The listing builds one solid part. Answer for the finished solid, in the listing's coordinates (mm). A direction names the side the tool comes from. Round coordinates to 2 decimals unless told otherwise and drop trailing zeros. Write each loop counter-clockwise with the first axis right and the second up, starting at its lowest first coordinate (ties: lowest second). Pieces come first, ordered by that corner, then holes. Notation, with made-up numbers: (86, 66) - (131, 66) arc R20 ccw to (131, 100) - close; hole circle Ø11 at (16, 6.5). An arc over 180 degrees is marked (long way). Answer in a Markdown table with one row per item.
from build123d import *

# Parameters (mm, degrees)
BOSS_EXTRUDE3_DEPTH   = 8
BOSS_EXTRUDE3_2_DEPTH = 8
SKETCH4_W             = 11
SKETCH4_H             = 10.5
BOSS_EXTRUDE4_DEPTH   = 2
FILLET3_R             = 3
MIRROR2_START         = -2
MIRROR2_DEPTH         = 10
MIRROR2_2_DEPTH       = 2
CHAMFER1_SIZE         = 2
FILLET4_R             = 4
FILLET5_R             = 2


# Read off the part's stored shape, not the designer's step: Mirror2
with BuildPart() as part:
    # Sketch3 → Boss-Extrude3 (new body)
    with BuildSketch(Plane(origin=(0, 0, 0), x_dir=(1, 0, 0), z_dir=(0, 1, 0))):
        with BuildLine():
            Line((-1.1, -5.25), (5.5, -5.25))
            Line((5.5, -5.25), (5.5, 5.25))
            Line((5.5, 5.25), (-5.5, 5.25))
            Line((-5.5, 5.25), (-5.5, -5.25))
            Line((-5.5, -5.25), (-3.5, -5.25))
            Line((-3.5, -5.25), (-3.5, 0.751))
            ThreePointArc((-3.5, 0.751), (0.5, 4.751), (4.5, 0.751))
            Line((4.5, 0.751), (4.5, 0.75))
            ThreePointArc((4.5, 0.75), (2.69089023, -2.596640106), (-1.1, -2.916060556))
            Line((-1.1, -2.916060556), (-1.1, -5.25))
        make_face()
    extrude(amount=BOSS_EXTRUDE3_DEPTH)



with BuildPart() as body_2:
    # Sketch3 → Boss-Extrude3 2 (new body)
    with BuildSketch(Plane(origin=(0, 0, 0), x_dir=(1, 0, 0), z_dir=(0, 1, 0))):
        with BuildLine():
            ThreePointArc((-1.7, 0.75), (0.5, -1.45), (2.7, 0.75))
            Line((2.7, 0.75), (2.7, 0.751))
            ThreePointArc((2.7, 0.751), (0.5, 2.951), (-1.7, 0.751))
            Line((-1.7, 0.751), (-1.7, 0.75))
        make_face()
    extrude(amount=BOSS_EXTRUDE3_2_DEPTH)


with BuildPart() as part_1:
    add(part.part)

    add(body_2.part)  # Boss-Extrude4 merges body 2
    # Sketch4 → Boss-Extrude4 (add)
    with BuildSketch(Plane(origin=(0, 0, 0), x_dir=(-1, 0, 0), z_dir=(0, -1, 0))):
        Rectangle(SKETCH4_W, SKETCH4_H)
    extrude(amount=BOSS_EXTRUDE4_DEPTH)

    # Fillet3
    # the kernel refuses this fillet: 3 mm, written as the material it takes off along each edge
    with BuildSketch(Plane(origin=(-1.1, 0, 2.916060556), x_dir=(1.3123233716119625e-12, 0, 1.0), z_dir=(0, 1, 0))) as fillet3_piece_1:
        with BuildLine():
            CenterArc((3.21838304, 2.866663483), FILLET3_R, 190.425211714, 62.42837206)
            ThreePointArc((0.267907213, 2.323807705), (0.307618872, 1.141882326), (0, 0))
            Line((0, 0), (2.333939444, 0))
        make_face()
    extrude(amount=13.847999938, mode=Mode.SUBTRACT)

    # Mirror2 outline → Mirror2 (add)
    with BuildSketch(Plane(origin=(0, 0, 0), x_dir=(1, 0, 0), z_dir=(0, 1, 0)).offset(MIRROR2_START)):
        with BuildLine():
            ThreePointArc((1.223807705, 13.683967769), (3.573697352, 12.309762604), (4.5, 9.75))
            Line((4.5, 9.75), (4.5, 9.749))
            ThreePointArc((4.5, 9.749), (0.5, 5.749), (-3.5, 9.749))
            Line((-3.5, 9.749), (-3.5, 15.75))
            Line((-3.5, 15.75), (-5.5, 15.75))
            Line((-5.5, 15.75), (-5.5, 5.25))
            Line((-5.5, 5.25), (5.5, 5.25))
            Line((5.5, 5.25), (5.5, 15.75))
            Line((5.5, 15.75), (-1.1, 15.75))
            ThreePointArc((-1.1, 15.75), (-0.226657287, 14.392419442), (1.223807705, 13.683967769))
        make_face()
        with BuildLine():
            ThreePointArc((-1.7, 9.749), (0.5, 7.549), (2.7, 9.749))
            Line((2.7, 9.749), (2.7, 9.75))
            ThreePointArc((2.7, 9.75), (0.5, 11.95), (-1.7, 9.75))
            Line((-1.7, 9.75), (-1.7, 9.749))
        make_face()
    extrude(amount=MIRROR2_DEPTH)

    # Mirror2 2 outline → Mirror2 2 (add)
    with BuildSketch(Plane(origin=(0, 0, 0), x_dir=(1, 0, 0), z_dir=(0, 1, 0)).offset(MIRROR2_START)):
        with BuildLine():
            Line((4.5, 9.749), (4.5, 9.75))
            ThreePointArc((4.5, 9.75), (3.573697352, 12.309762604), (1.223807705, 13.683967769))
            ThreePointArc((1.223807705, 13.683967769), (-0.226657287, 14.392419442), (-1.1, 15.75))
            Line((-1.1, 15.75), (-3.5, 15.75))
            Line((-3.5, 15.75), (-3.5, 9.749))
            ThreePointArc((-3.5, 9.749), (0.5, 5.749), (4.5, 9.749))
        make_face()
        with BuildLine():
            Line((2.7, 9.75), (2.7, 9.749))
            ThreePointArc((2.7, 9.749), (0.5, 7.549), (-1.7, 9.749))
            Line((-1.7, 9.749), (-1.7, 9.75))
            ThreePointArc((-1.7, 9.75), (0.5, 11.95), (2.7, 9.75))
        make_face(mode=Mode.SUBTRACT)
    extrude(amount=MIRROR2_2_DEPTH)

    # Chamfer1
    # the kernel refuses this chamfer: 2 mm, written as the material it adds along each edge
    with BuildSketch(Plane(origin=(0.5, 0, -9.749), x_dir=(1, 0, 0), z_dir=(0, 0, -1))) as chamfer1_piece_1:
        Polygon((2.2 + CHAMFER1_SIZE, 0), (2.2, -CHAMFER1_SIZE), (2.2, 0), align=None)
    revolve(axis=Axis((0.5, 0, -9.749), (0, -1, 0)), revolution_arc=180)
    with BuildSketch(Plane(origin=(-1.7, 0, -9.749), x_dir=(-0.9996219169112968, -0.027495876610586365, 0), z_dir=(0, 0, -1)), Plane(origin=(2.7, 0, -9.75), x_dir=(0.9996219169112968, -0.027495876610586365, 0), z_dir=(0, 0, 1))) as chamfer1_piece_2:
        Polygon((CHAMFER1_SIZE * 0.999621916911, CHAMFER1_SIZE * 0.0274958766106), (-CHAMFER1_SIZE * 0.0274958766106, CHAMFER1_SIZE * 0.999621916911), (0, 0), align=None)
    extrude(amount=0.001)
    with BuildSketch(Plane(origin=(0.5, 0, -9.75), x_dir=(-1, 0, 0), z_dir=(0, 0, 1))) as chamfer1_piece_3:
        Polygon((2.2 + CHAMFER1_SIZE, 0), (2.2, -CHAMFER1_SIZE), (2.2, 0), align=None)
    revolve(axis=Axis((0.5, 0, -9.75), (0, -1, 0)), revolution_arc=180)
    with BuildSketch(Plane(origin=(0.5, 0, -0.751), x_dir=(1, 0, 0), z_dir=(0, 0, 1))) as chamfer1_piece_4:
        Polygon((2.2 + CHAMFER1_SIZE, 0), (2.2, CHAMFER1_SIZE), (2.2, 0), align=None)
    revolve(axis=Axis((0.5, 0, -0.751), (0, 1, 0)), revolution_arc=180)
    with BuildSketch(Plane(origin=(-1.7, 0, -0.751), x_dir=(-0.9996219169112968, -0.027495876610586372, 0), z_dir=(0, 0, 1)), Plane(origin=(2.7, 0, -0.75), x_dir=(0.9996219169112968, -0.027495876610586358, 0), z_dir=(0, 0, -1))) as chamfer1_piece_5:
        Polygon((CHAMFER1_SIZE * 0.999621916911, -CHAMFER1_SIZE * 0.0274958766106), (-CHAMFER1_SIZE * 0.0274958766106, -CHAMFER1_SIZE * 0.999621916911), (0, 0), align=None)
    extrude(amount=0.001)
    with BuildSketch(Plane(origin=(0.5, 0, -0.75), x_dir=(-1, 0, 0), z_dir=(0, 0, -1))) as chamfer1_piece_6:
        Polygon((2.2 + CHAMFER1_SIZE, 0), (2.2, CHAMFER1_SIZE), (2.2, 0), align=None)
    revolve(axis=Axis((0.5, 0, -0.75), (0, 1, 0)), revolution_arc=180)

    # Fillet4
    fillet4_edges = [part_1.edges().sort_by_distance(p)[0] for p in [
        (5.5, 3, 5.25),
        (5.5, 3, -15.75),
    ]]
    fillet(fillet4_edges, radius=FILLET4_R)

    # Fillet5
    fillet5_edges = [part_1.edges().sort_by_distance(p)[0] for p in [
        (-5.5, 3, -15.75),
        (-5.5, 3, 5.25),
    ]]
    fillet(fillet5_edges, radius=FILLET5_R)


solid = part_1.part
(1) Section A-A (y = 6.5) is taken. State how many separate pieces and enclosed holes the cut face has, and give its area (3 significant figures).
Checked values:
| item | result |
|---|---|
| separate pieces | 3 |
| enclosed holes | 0 |
| area | 133 mm2 |
(2) Find the intervals of material crossed by line 1 (X direction, y = 2.75, z = -1.5); line 2 (X direction, y = 0.5, z = -0.25); line 3 (Z direction, x = 0.75, y = 4), in increasing order.
Checked values:
| item | result |
|---|---|
| line 1 | x = -5.5 to -3.43, -1.57 to 2.57, 4.43 to 5.5 |
| line 2 | x = -5.5 to -3.5, -3.17 to 4.17, 4.47 to 5.5 |
| line 3 | z = -15.75 to -13.81, -11.94 to -7.56, -5.76 to -4.74, -2.94 to 1.44, 3.31 to 5.25 |
(3) Section D-D (x = 4.75) is taken. Give the vertices of the cut face in (y, z).
Checked values:
| item | result |
|---|---|
| outline | (-2, -14.08) - (8, -14.08) - (8, 3.58) - (-2, 3.58) - close |
(4) For a pull along Z with two mould halves and no side action, classify faces 1 (the flat face through (0, -2, -5)), 2 (the cylindrical face through (0.55, 4.96, -11.95)), 3 (the cylindrical face through (-4.9, 2.93, 4.68)), 4 (the cylindrical face through (4.297, 3.07, -14.609)) as pulls with the +Z half, pulls with the -Z half, needs draft (parallel to the pull), parting line crosses it, or undercut.
Checked values:
| item | result |
|---|---|
| face 1 | needs draft |
| face 2 | undercut |
| face 3 | pulls with the +Z half |
| face 4 | pulls with the -Z half |
(5) For faces 5 (the flat face through (-3.5, 4, 2)), 6 (the flat face through (-5.5, 3, -5)), 7 (the cylindrical face through (0.55, 4.96, -2.95)), determine the directions among +Z, -Z, +X, -X, +Y, -Y from which every point of the face is accessible in a straight line to the end or side of a thin tool.
Checked values:
| item | result |
|---|---|
| face 5 | +Z, +Y |
| face 6 | +Z, -Z, -X, +Y, -Y |
| face 7 | +Y |
(6) A flat-ended cylindrical pin translates along its axis: pin 1 (3 mm diameter, centred on x = 4, y = 5.5, fed in from -Z). Find the tip coordinate at first contact, or state that the pin passes through.
Checked values:
| item | result |
|---|---|
| pin 1 | stops at z = -15.62 |
(7) Section C-C (z = -14.25) is taken. Give the vertices of the cut face in (x, y), and give its area (3 significant figures).
Checked values:
| item | result |
|---|---|
| outline | (-5.44, -2) - (4.62, -2) - (4.62, 8) - (-0.05, 8) - (-0.05, 0) - (-3.5, 0) - (-3.5, 8) - (-5.44, 8) - close |
| area | 73.0 mm2 |
